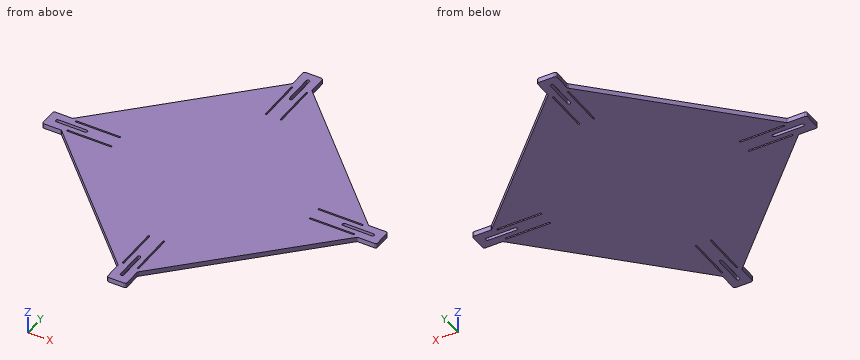
Autodesk Inventor part; units mm, degrees
ref_plane "YZ Plane" through (0, 0, 0) normal (1, 0, 0) x (0, 1, 0)
ref_plane "XZ Plane" through (0, 0, 0) normal (0, 1, 0) x (-1, 0, 0)
ref_plane "XY Plane" through (0, 0, 0) normal (0, 0, 1) x (1, 0, 0)
sketch "Sketch2" plane through (0, 0, 0) normal (0, 0, 1) x (1, 0, 0)
  circle A0 centre (0, 0) radius 327.5 construction
  line L0 (260.6, -21.1) -> (302.8, -21.1) construction
  line L1 (302.8, -21.1) -> (302.8, 21.1) construction
  line L2 (302.8, 21.1) -> (260.6, 21.1) construction
  line L3 (260.6, 21.1) -> (260.6, -21.1) construction
  line L4 (260.6, -21.1) -> (302.8, 21.1) construction
  line L5 (302.8, -21.1) -> (260.6, 21.1) construction
  line L6 (297.2, 15.5) -> (207.0955, 15.5) construction
  line L7 (297.2, 17.1) -> (207.0955, 17.1)
  line L8 (207.0955, 13.9) -> (297.2, 13.9)
  arc A1 (297.2, 13.9) -> (297.2, 17.1) centre (297.2, 15.5) ccw
  arc A2 (207.0955, 17.1) -> (207.0955, 13.9) centre (207.0955, 15.5) ccw
  line L9 (297.2, -15.5) -> (207.0955, -15.5) construction
  line L10 (297.2, -13.9) -> (207.0955, -13.9)
  line L11 (207.0955, -17.1) -> (297.2, -17.1)
  arc A3 (297.2, -17.1) -> (297.2, -13.9) centre (297.2, -15.5) ccw
  arc A4 (207.0955, -13.9) -> (207.0955, -17.1) centre (207.0955, -15.5) ccw
  line L12 (327.5, 0) -> (268.3955, 0) construction
  line L13 (327.5, 3.4) -> (268.3955, 3.4)
  line L14 (268.3955, -3.4) -> (327.5, -3.4)
  arc A5 (327.5, -3.4) -> (327.5, 3.4) centre (327.5, 0) ccw
  arc A6 (268.3955, 3.4) -> (268.3955, -3.4) centre (268.3955, 0) ccw
  line L15 (307.5, -20) -> (347.5, -20)
  line L16 (347.5, -20) -> (347.5, 20)
  line L17 (347.5, 20) -> (307.5, 20)
  line L18 (307.5, 20) -> (307.5, -20)
  line L19 (307.5, -20) -> (347.5, 20) construction
  line L20 (347.5, -20) -> (307.5, 20) construction
  circle A7 centre (327.5, 0) radius 3.4
  arc A8 (-3.4, 268.3955) -> (3.4, 268.3955) centre (0, 268.3955) ccw
  line L21 (-13.9, 207.0955) -> (-13.9, 297.2)
  line L22 (-17.1, 297.2) -> (-17.1, 207.0955)
  line L23 (-15.5, 297.2) -> (-15.5, 207.0955) construction
  line L24 (17.1, 207.0955) -> (17.1, 297.2)
  line L25 (15.5, 297.2) -> (15.5, 207.0955) construction
  line L26 (13.9, 297.2) -> (13.9, 207.0955)
  arc A9 (-17.1, 207.0955) -> (-13.9, 207.0955) centre (-15.5, 207.0955) ccw
  arc A10 (13.9, 207.0955) -> (17.1, 207.0955) centre (15.5, 207.0955) ccw
  line L27 (21.1, 302.8) -> (-21.1, 302.8) construction
  arc A11 (-13.9, 297.2) -> (-17.1, 297.2) centre (-15.5, 297.2) ccw
  arc A12 (17.1, 297.2) -> (13.9, 297.2) centre (15.5, 297.2) ccw
  line L28 (0, 327.5) -> (0, 268.3955) construction
  line L29 (-3.4, 327.5) -> (-3.4, 268.3955)
  line L30 (3.4, 268.3955) -> (3.4, 327.5)
  line L31 (21.1, 260.6) -> (21.1, 302.8) construction
  line L32 (21.1, 302.8) -> (-21.1, 260.6) construction
  line L33 (-21.1, 260.6) -> (21.1, 260.6) construction
  line L34 (21.1, 260.6) -> (-21.1, 302.8) construction
  line L35 (-21.1, 302.8) -> (-21.1, 260.6) construction
  line L36 (-20, 307.5) -> (20, 307.5)
  arc A13 (3.4, 327.5) -> (-3.4, 327.5) centre (0, 327.5) ccw
  circle A14 centre (0, 327.5) radius 3.4
  line L37 (20, 307.5) -> (20, 347.5)
  line L38 (-20, 347.5) -> (-20, 307.5)
  line L39 (20, 307.5) -> (-20, 347.5) construction
  line L40 (20, 347.5) -> (-20, 307.5) construction
  line L41 (20, 347.5) -> (-20, 347.5)
  arc A15 (-268.3955, -3.4) -> (-268.3955, 3.4) centre (-268.3955, 0) ccw
  line L42 (-207.0955, -13.9) -> (-297.2, -13.9)
  line L43 (-297.2, -17.1) -> (-207.0955, -17.1)
  line L44 (-297.2, -15.5) -> (-207.0955, -15.5) construction
  line L45 (-207.0955, 17.1) -> (-297.2, 17.1)
  line L46 (-297.2, 15.5) -> (-207.0955, 15.5) construction
  line L47 (-297.2, 13.9) -> (-207.0955, 13.9)
  arc A16 (-207.0955, -17.1) -> (-207.0955, -13.9) centre (-207.0955, -15.5) ccw
  arc A17 (-207.0955, 13.9) -> (-207.0955, 17.1) centre (-207.0955, 15.5) ccw
  line L48 (-302.8, 21.1) -> (-302.8, -21.1) construction
  arc A18 (-297.2, -13.9) -> (-297.2, -17.1) centre (-297.2, -15.5) ccw
  arc A19 (-297.2, 17.1) -> (-297.2, 13.9) centre (-297.2, 15.5) ccw
  line L49 (-327.5, 0) -> (-268.3955, 0) construction
  line L50 (-327.5, -3.4) -> (-268.3955, -3.4)
  line L51 (-268.3955, 3.4) -> (-327.5, 3.4)
  line L52 (-260.6, 21.1) -> (-302.8, 21.1) construction
  line L53 (-302.8, 21.1) -> (-260.6, -21.1) construction
  line L54 (-260.6, -21.1) -> (-260.6, 21.1) construction
  line L55 (-260.6, 21.1) -> (-302.8, -21.1) construction
  line L56 (-302.8, -21.1) -> (-260.6, -21.1) construction
  line L57 (-307.5, -20) -> (-307.5, 20)
  arc A20 (-327.5, 3.4) -> (-327.5, -3.4) centre (-327.5, 0) ccw
  circle A21 centre (-327.5, 0) radius 3.4
  line L58 (-307.5, 20) -> (-347.5, 20)
  line L59 (-347.5, -20) -> (-307.5, -20)
  line L60 (-307.5, 20) -> (-347.5, -20) construction
  line L61 (-347.5, 20) -> (-307.5, -20) construction
  line L62 (-347.5, 20) -> (-347.5, -20)
  arc A22 (3.4, -268.3955) -> (-3.4, -268.3955) centre (0, -268.3955) ccw
  line L63 (13.9, -207.0955) -> (13.9, -297.2)
  line L64 (17.1, -297.2) -> (17.1, -207.0955)
  line L65 (15.5, -297.2) -> (15.5, -207.0955) construction
  line L66 (-17.1, -207.0955) -> (-17.1, -297.2)
  line L67 (-15.5, -297.2) -> (-15.5, -207.0955) construction
  line L68 (-13.9, -297.2) -> (-13.9, -207.0955)
  arc A23 (17.1, -207.0955) -> (13.9, -207.0955) centre (15.5, -207.0955) ccw
  arc A24 (-13.9, -207.0955) -> (-17.1, -207.0955) centre (-15.5, -207.0955) ccw
  line L69 (-21.1, -302.8) -> (21.1, -302.8) construction
  arc A25 (13.9, -297.2) -> (17.1, -297.2) centre (15.5, -297.2) ccw
  arc A26 (-17.1, -297.2) -> (-13.9, -297.2) centre (-15.5, -297.2) ccw
  line L70 (0, -327.5) -> (0, -268.3955) construction
  line L71 (3.4, -327.5) -> (3.4, -268.3955)
  line L72 (-3.4, -268.3955) -> (-3.4, -327.5)
  line L73 (-21.1, -260.6) -> (-21.1, -302.8) construction
  line L74 (-21.1, -302.8) -> (21.1, -260.6) construction
  line L75 (21.1, -260.6) -> (-21.1, -260.6) construction
  line L76 (-21.1, -260.6) -> (21.1, -302.8) construction
  line L77 (21.1, -302.8) -> (21.1, -260.6) construction
  line L78 (20, -307.5) -> (-20, -307.5)
  arc A27 (-3.4, -327.5) -> (3.4, -327.5) centre (0, -327.5) ccw
  circle A28 centre (0, -327.5) radius 3.4
  line L79 (-20, -307.5) -> (-20, -347.5)
  line L80 (20, -347.5) -> (20, -307.5)
  line L81 (-20, -307.5) -> (20, -347.5) construction
  line L82 (-20, -347.5) -> (20, -307.5) construction
  line L83 (-20, -347.5) -> (20, -347.5)
  line L84 (-20, 307.5) -> (-307.5, 20)
  line L85 (-307.5, -20) -> (-20, -307.5)
  line L86 (307.5, -20) -> (20, -307.5)
  line L87 (20, 307.5) -> (307.5, 20)
  point P0 (281.7, 0)
  point P1 (252.1478, 15.5)
  point P2 (252.1478, -15.5)
  point P3 (297.9478, 0)
  point P4 (15.5, 252.1478)
  point P5 (0, 281.7)
  point P6 (-15.5, 252.1478)
  point P7 (0, 297.9478)
  point P8 (-252.1478, 15.5)
  point P9 (-281.7, 0)
  point P10 (-252.1478, -15.5)
  point P11 (-297.9478, 0)
  point P12 (-15.5, -252.1478)
  point P13 (0, -281.7)
  point P14 (15.5, -252.1478)
  point P15 (0, -297.9478)
  dimension "d26" = 655
  dimension "d110" = 42.2
  dimension "d113" = 42.2
  dimension "d114" = 3.2
  dimension "d115" = 90.1045
  dimension "d116" = 5.6
  dimension "d117" = 3.2
  dimension "d118" = 5.6
  dimension "d119" = 90.1045
  dimension "d122" = 59.1045
  dimension "d123" = 6.8
  dimension "d134" = 40
  dimension "d135" = 40
  dimension "d136" = 6.8
  dimension "d137" = 327.5
  dimension "d138" = 4.7
  dimension "d141" = 360
extrude "Extrusion9" add sketch "Sketch2" against normal blind 10 contours L13 L18 L17 L16 L15 L14 A5 | L13 A6 L14 L18 L86 L78 L71 A22 L72 L85 L57 L50 A15 L51 L84 L36 L29 A8 L30 L87 | L36 L30 A13 L29 L38 L41 L37 | L80 L83 L79 L78 L72 A27 L71 | L57 L51 A20 L50 L59 L62 L58
fillet "Fillet7" radius 4 16 edges at (20, 347.5, -5) (20, 307.5, -5) (-20, 347.5, -5) (-20, 307.5, -5) (-347.5, 20, -5) (-307.5, 20, -5) (-347.5, -20, -5) (-307.5, -20, -5) (-20, -347.5, -5) (-20, -307.5, -5) (347.5, -20, -5) (20, -347.5, -5) (307.5, 20, -5) (347.5, 20, -5) (20, -307.5, -5) (307.5, -20, -5)
equation "\"d26\" = ring_outer_diam + bar_width"
equation "\"ring_inner_diam\" = 565"
equation "\"bar_width\" = 40"
equation "\"bar_hole_diam\" = 6.8"
equation "\"ring_outer_diam\" = 615"
equation "\"motor_width\" = 42.2"
equation "\"dist_motor_bar\" = 4.7"
equation "\"motor_slot_diam\" = 3.2"
equation "\"motor_hole_edge_dist\" = 5.6"
equation "\"motor_slot_length\" = 90.1045"
equation "\"bar_slot_diam\" = 6.8"
equation "\"bar_slot_length\" = 59.1045"
equation "\"dist_motor_holes\" = 31"
equation "\"diag_dist_bar_holes_old_fridge\" = 536.791"
properties part number "base_plate" material "Aluminum 6061"
Work out the finished part from the listing and answer in its coordinate system (mm). Round coordinates to 2 decimals unless told otherwise and drop trailing zeros. Order: outer loops, then holes, each group sorted by start corner. A loop starts at its lowest first (then second) coordinate and runs counter-clockwise, first axis right, second up. Notation, with made-up numbers: M -18,21.5 L 34,21.5 A28 ccw 34,52.5 Z; hole C 4.25,-15 d1. An arc over 180 degrees is marked long. Put each result on its own line as item: value. Start each with the question number.
Q1. Section B-B, the plane z = -5 is taken. Give the number of separate pieces and of enclosed holes in the cut face, and give its area (3 significant figures).
Q2. Section C-C, the plane y = 64 is taken. Write down the section's boundary in (x, z), and give its area (3 significant figures).
Q3. Section D-D, the plane x = 127 is taken. Write down the section's boundary in (y, z), and give its area (3 significant figures).
Q4. Straight lines are drawn through the part: L1, parallel to X at y = 242, z = -9; L2, parallel to Y at x = -264, z = -1.25; L3, parallel to Y at x = -286, z = -1. For each, find the intervals that lie inside material, in ascending order. Write a range as [from, to].
Q5. Section A-A, the plane x = 216 is taken. Write down the section's boundary in (y, z).
Q6. Flat-ended cylindrical pins translate along their axes: pin 1 (5 mm diameter, centred on x = 293, z = -2.5, fed in from +Y); pin 2 (4 mm diameter, centred on x = -55.5, z = -1, fed in from -Y); pin 3 (2 mm diameter, centred on x = 233.5, z = -8.5, fed in from -Y). Find the tip coordinate at first contact, or state that the pin passes through.
Findings below:
1. separate pieces: 1
1. enclosed holes: 12
1. area: 215,000 mm^2
2. outline: M -263.5,-10 L 263.5,-10 L 263.5,0 L -263.5,0 Z
2. area: 5,270 mm^2
3. outline: M -200.5,-10 L 200.5,-10 L 200.5,0 L -200.5,0 Z
3. area: 4,010 mm^2
4. L1: x = [-85.5, -17.1], [-13.9, 13.9], [17.1, 85.5]
4. L2: y = [-63.5, -17.1], [-13.9, 13.9], [17.1, 63.5]
4. L3: y = [-41.5, -17.1], [-13.9, -3.4], [3.4, 13.9], [17.1, 41.5]
5. outline: M -111.5,-10 L -17.1,-10 L -17.1,0 L -111.5,0 Z; M -13.9,-10 L 13.9,-10 L 13.9,0 L -13.9,0 Z; M 17.1,-10 L 111.5,-10 L 111.5,0 L 17.1,0 Z
6. pin 1: stops at y = 37
6. pin 2: stops at y = -274
6. pin 3: stops at y = -95
